Source: CAD feature listing. Evaluate the final solid. Frame: model axes, mm. A direction names the side the tool comes from. Round coordinates to 2 decimals unless told otherwise and drop trailing zeros. Write each loop counter-clockwise with the first axis right and the second up, starting at its lowest first coordinate (ties: lowest second). Pieces come first, ordered by that corner, then holes.
from build123d import *

# Parameters (mm, degrees)
SKETCH1_R           = 15.875
BOSS_EXTRUDE1_DEPTH = 25.4
SKETCH2_R           = 5.715
CUT_EXTRUDE1_DEPTH  = 34.89972345
SKETCH3_R           = 6.985
CUT_EXTRUDE2_DEPTH  = 1.27
CIRPATTERN3_COUNT   = 2
CIRPATTERN4_COUNT   = 3
CIRPATTERN5_COUNT   = 2


with BuildPart() as part:
    # Sketch1 → Boss-Extrude1 (new body)
    with BuildSketch(Plane(origin=(0, 0, 0), x_dir=(1, 0, 0), z_dir=(0, 1, 0))):
        with Locations(Location((0, 0, 0), (0, 0, 90))):
            Circle(SKETCH1_R)
    extrude(amount=BOSS_EXTRUDE1_DEPTH)

    # Sketch2 → Cut-Extrude1 (cut, through all)
    with BuildSketch(Plane(origin=(0, 25.4, 0), x_dir=(1, 0, 0), z_dir=(0, 1, 0))):
        with Locations(Location((0, 0, 0), (0, 0, 270))):
            Circle(SKETCH2_R)
    extrude(amount=-CUT_EXTRUDE1_DEPTH, mode=Mode.SUBTRACT)

    # Sketch3 → Cut-Extrude2 (cut)
    with BuildSketch(Plane(origin=(0, 25.4, 0), x_dir=(1, 0, 0), z_dir=(0, 1, 0))):
        with Locations(Location((0, 0, 0), (0, 0, 270))):
            Circle(SKETCH3_R)
    extrude(amount=-CUT_EXTRUDE2_DEPTH, mode=Mode.SUBTRACT)

    # Sketch10 → 1/4 (0.25) Diameter Hole2 (revolve, cut)
    with BuildSketch(Plane(origin=(8.917384444, 0, 6.43673099), x_dir=(0, 0, -1), z_dir=(1, 0, 0))):
        Polygon((0, 0), (0, 20.957732465), (3.175, 19.05), (3.175, 0), align=None)
    f_1_4_0_25_diameter_hole2 = revolve(axis=Axis((8.917384444, -6.35, 6.43673099), (0, 1, 0)), mode=Mode.SUBTRACT)

    # CirPattern3: 1/4 (0.25) Diameter Hole2 ×2 about axis
    cirpattern3_axis = Axis((0, 0, 0), (0, 1, 0))
    for i in range(1, CIRPATTERN3_COUNT):
        add(f_1_4_0_25_diameter_hole2.rotate(cirpattern3_axis, i * 360 / CIRPATTERN3_COUNT), mode=Mode.SUBTRACT)

    # Sketch13 → 5/64 (0.07813) Diameter Hole1 (revolve, cut)
    with BuildSketch(Plane(origin=(-5.914180419, 25.4, -9.780969787), x_dir=(0, 0, 1), z_dir=(1, 0, 0))):
        Polygon((0, 0), (0, 10.75620455), (0.992251, 10.16), (0.992251, 0.532828266), (1.627251, 0), align=None)
    f_5_64_0_07813_diameter_hole1 = revolve(axis=Axis((-5.914180419, 31.75, -9.780969787), (0, -1, 0)), mode=Mode.SUBTRACT)

    # CirPattern4: 5/64 (0.07813) Diameter Hole1 ×3 about axis
    cirpattern4_axis = Axis((0, 0, 0), (0, 1, 0))
    for i in range(1, CIRPATTERN4_COUNT):
        add(f_5_64_0_07813_diameter_hole1.rotate(cirpattern4_axis, i * 360 / CIRPATTERN4_COUNT), mode=Mode.SUBTRACT)

    # Sketch16 → 1/16 (0.0625) Diameter Hole1 (revolve, cut)
    with BuildSketch(Plane(origin=(-3.214022597, 0, -10.637561516), x_dir=(0, 0, -1), z_dir=(1, 0, 0))):
        Polygon((0, 0), (0, 13.176933116), (0.79375, 12.7), (0.79375, 0.532828266), (1.42875, 0), align=None)
    f_1_16_0_0625_diameter_hole1 = revolve(axis=Axis((-3.214022597, -6.35, -10.637561516), (0, 1, 0)), mode=Mode.SUBTRACT)

    # CirPattern5: 1/16 (0.0625) Diameter Hole1 ×2 about axis
    cirpattern5_axis = Axis((0, 0, 0), (0, 1, 0))
    for i in range(1, CIRPATTERN5_COUNT):
        add(f_1_16_0_0625_diameter_hole1.rotate(cirpattern5_axis, i * 360 / CIRPATTERN5_COUNT), mode=Mode.SUBTRACT)


solid = part.part
1) Material intervals for line 1 (X direction, y = 16.5, z = 4); line 2 (X direction, y = 12, z = 0) (3 decimals); line 3 (Z direction, x = -3.5, y = 2.5), sorted ascending.
Taken from the geometry:
line 1: x = -15.36 to -4.08, 4.08 to 6.88, 10.95 to 15.36
line 2: x = -15.875 to -5.715, 5.715 to 15.875
line 3: z = -15.48 to -11.38, -9.9 to -4.52, 4.52 to 15.48
2) Section query A-A on x = 0. Return the cut outline in (y, z) (3 decimals).
Taken from the geometry:
outline: (0, -15.875) - (25.4, -15.875) - (25.4, -6.985) - (24.13, -6.985) - (24.13, -5.715) - (0, -5.715) - close; (0, 5.715) - (24.13, 5.715) - (24.13, 6.985) - (25.4, 6.985) - (25.4, 15.875) - (0, 15.875) - close
3) Reachability of faces 4 (the face through (-6.24, 9.39, -4.73)), 5 (the face through (5.666, 12.234, -0.744)), 6 (the face through (-4.946, 20.121, -9.996)) from +Z, -Z, +X, -X, +Y, -Y: full face, straight path, thin tool, end or side. Return the list, or none.
Taken from the geometry:
face 4: -Y
face 5: +Y, -Y
face 6: +Y
4) Pull-direction query (X, two-part tool) for faces 1 (the face through (0, 0, -7)), 2 (the face through (0, 24.13, -6)), 3 (the face through (15.497, 12.522, 3.441)); classes: released by +X, released by -X, zero draft, split by the parting line, or undercut.
Taken from the geometry:
face 1: zero draft
face 2: undercut
face 3: split by the parting line
5) Section query B-B on y = 19.5. State how many separate pieces and enclosed holes the cut face has, then the cut area to 3 significant figures.
Taken from the geometry:
separate pieces: 1
enclosed holes: 6
area: 643 mm2
6) Contact query for flat-ended pins moving along their axis: P1, Ø10, axis at y = 19.5, z = 9.5, coming from the +X side; P2, Ø1.5, axis at y = 22, z = 9.5, coming from the +X side; P3, Ø1.2, axis at x = 11.43, z = -0.23, coming from the +Y side; P4, Ø10.5, axis at x = 0, z = 0, coming from the -Y side. Output: stop coordinate, or through.
Taken from the geometry:
P1: stops at x = 15.22
P2: stops at x = 13.25
P3: stops at y = 15.01
P4: passes through
